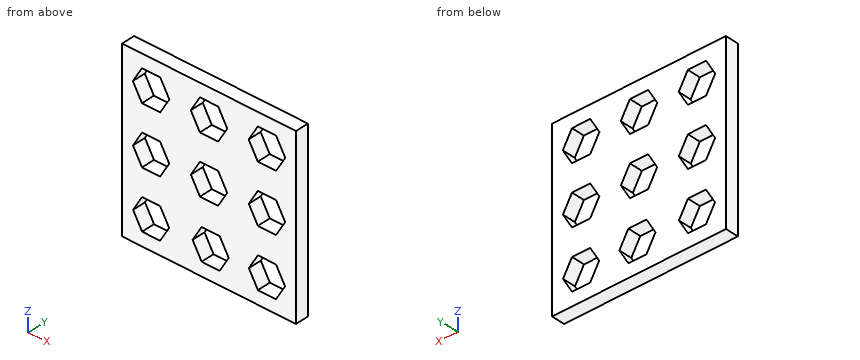
```python
from build123d import *

# Parameters (mm, degrees)
SKETCH1_W           = 30
SKETCH1_H           = 30
BOSS_EXTRUDE1_DEPTH = 2.3
CUT_EXTRUDE3_DEPTH  = 2.3


with BuildPart() as part:
    # Sketch1 → Boss-Extrude1 (new body)
    with BuildSketch(Plane(origin=(0, 0, 0), x_dir=(1, 0, 0), z_dir=(0, 1, 0))):
        Rectangle(SKETCH1_W, SKETCH1_H)
    extrude(amount=BOSS_EXTRUDE1_DEPTH)

    # Sketch2 → Cut-Extrude3 (cut)
    with BuildSketch(Plane(origin=(0, 2.3, 0), x_dir=(1, 0, 0), z_dir=(0, 1, 0))):
        Polygon((3.135011962, 0), (1.567505981, 2.715), (-1.567505981, 2.715), (-3.135011962, 0), (-1.567505981, -2.715), (1.567505981, -2.715), align=None)
        Polygon((-6.888082049, 10), (-8.444041025, 12.695), (-11.555958975, 12.695), (-13.111917951, 10), (-11.555958975, 7.305), (-8.444041025, 7.305), align=None)
        Polygon((3.39878526, 10), (1.839939533, 12.7), (-1.277751921, 12.7), (-2.836597647, 10), (-1.277751921, 7.3), (1.839939533, 7.3), align=None)
        Polygon((13.122373208, 10), (11.56064073, 12.705), (8.437175774, 12.705), (6.875443295, 10), (8.437175774, 7.295), (11.56064073, 7.295), align=None)
        Polygon((13.139693716, 0), (11.569300984, 2.72), (8.42851552, 2.72), (6.858122787, 0), (8.42851552, -2.72), (11.569300984, -2.72), align=None)
        Polygon((13.157014224, -10), (11.577961238, -7.265), (8.419855266, -7.265), (6.840802279, -10), (8.419855266, -12.735), (11.577961238, -12.735), align=None)
        Polygon((3.15233247, -10), (1.576166235, -7.27), (-1.576166235, -7.27), (-3.15233247, -10), (-1.576166235, -12.73), (1.576166235, -12.73), align=None)
        Polygon((-6.853441033, -10), (-8.426720516, -7.275), (-11.573279484, -7.275), (-13.146558967, -10), (-11.573279484, -12.725), (-8.426720516, -12.725), align=None)
        Polygon((-6.870761541, 0), (-8.43538077, 2.71), (-11.56461923, 2.71), (-13.129238459, 0), (-11.56461923, -2.71), (-8.43538077, -2.71), align=None)
    extrude(amount=-CUT_EXTRUDE3_DEPTH, mode=Mode.SUBTRACT)


solid = part.part
```
Source: CAD feature listing. Evaluate the final solid. Frame: model axes, mm. Give positions to 0.01 mm unless a question says otherwise; leave off trailing zeros. Order: outer loops, then holes, each group sorted by start corner. A loop starts at its lowest first (then second) coordinate and runs counter-clockwise, first axis right, second up. Notation, with made-up numbers: (53, 77.5) -> (106, 77.5) arc R20 ccw to (106, 99.5) -> close; hole circle Ø4 at (43, 37.25). An arc over 180 degrees is marked (long way). Use a Markdown table: item, result.
Q1. Section A-A (x = -9.25). Return the cut outline in (y, z) (3 decimals), and give its area (3 significant figures).
A:
| item | result |
|---|---|
| outline | (0, -15) -> (2.3, -15) -> (2.3, -12.695) -> (0, -12.695) -> close; (0, -7.305) -> (2.3, -7.305) -> (2.3, -2.71) -> (0, -2.71) -> close; (0, 2.71) -> (2.3, 2.71) -> (2.3, 7.275) -> (0, 7.275) -> close; (0, 12.725) -> (2.3, 12.725) -> (2.3, 15) -> (0, 15) -> close |
| area | 31.6 mm^2 |
Q2. Material intervals for line 1 (Z direction, x = -11.25, y = 1.5) (3 decimals); line 2 (X direction, y = 1.3, z = -8.5); line 3 (Z direction, x = -2, y = 1.75), sorted ascending. Write a range as [from, to].
A:
| item | result |
|---|---|
| line 1 | [-15, -12.695], [-7.305, -2.71], [2.71, 7.275], [12.725, 15] |
| line 2 | [-15, -12.25], [-7.75, -1.97], [2.53, 7.74], [12.26, 15] |
| line 3 | [-15, -11.45], [-8.55, -1.97], [1.97, 8], [12, 15] |
Q3. Section C-C (y = 0.45). State how many separate pieces and enclosed holes the cut face has, and give its area (3 significant figures).
A:
| item | result |
|---|---|
| separate pieces | 1 |
| enclosed holes | 9 |
| area | 670 mm^2 |
Q4. Section B-B (x = -0.25). Return the cut outline in (y, z) (3 decimals).
A:
| item | result |
|---|---|
| outline | (0, -15) -> (2.3, -15) -> (2.3, -12.7) -> (0, -12.7) -> close; (0, -7.3) -> (2.3, -7.3) -> (2.3, -2.715) -> (0, -2.715) -> close; (0, 2.715) -> (2.3, 2.715) -> (2.3, 7.27) -> (0, 7.27) -> close; (0, 12.73) -> (2.3, 12.73) -> (2.3, 15) -> (0, 15) -> close |
